```python
from build123d import *

# Parameters (mm, degrees)
SKETCH_1_R               = 37.5
EXTRUDE_1_DEPTH          = 7.5
SKETCH_2_R               = 2.05
CUT_EXTRUDE_1_DEPTH      = 54.560713214
CUT_EXTRUDE_2_DEPTH      = 3
PATTERN_CIRCULAR_1_COUNT = 4
SKETCH_4_R               = 3.05
CUT_EXTRUDE_3_DEPTH      = 4.5
PATTERN_CIRCULAR_2_COUNT = 6
SKETCH_7_R               = 28.2
SKETCH_7_R_2             = 21
CUT_EXTRUDE_4_DEPTH      = 4
SKETCH_9_R               = 6
CUT_EXTRUDE_5_DEPTH      = 54.560713214
EXTRUDE_3_DEPTH          = 4
FILLET_1_R               = 3
FILLET_3_R               = 3
FILLET_5_R               = 3.5
FILLET_6_R               = 3.5


with BuildPart() as part:
    # 草图1 → 凸台-拉伸1 (new body)
    with BuildSketch(Plane(origin=(0, 0, 0), x_dir=(1, 0, 0), z_dir=(0, 1, 0))):
        with Locations(Location((0, 0, 0), (0, 0, 270))):
            Circle(SKETCH_1_R)
    extrude(amount=EXTRUDE_1_DEPTH)

    # 草图2 → 切除-拉伸1 (cut, through all)
    with BuildSketch(Plane(origin=(0, 7.5, 0), x_dir=(1, 0, 0), z_dir=(0, 1, 0))):
        with Locations(Location((-31.5, 0, 0), (0, 0, 270))):
            Circle(SKETCH_2_R)
    cut_extrude_1 = extrude(amount=-CUT_EXTRUDE_1_DEPTH, mode=Mode.SUBTRACT)

    # 草图3 → 切除-拉伸2 (cut)
    with BuildSketch(Plane(origin=(0, 7.5, 0), x_dir=(1, 0, 0), z_dir=(0, 1, 0))):
        Polygon((-31.5, 3.944), (-34.915604193, 1.972), (-34.915604193, -1.972), (-31.5, -3.944), (-28.084395807, -1.972), (-28.084395807, 1.972), align=None)
    cut_extrude_2 = extrude(amount=-CUT_EXTRUDE_2_DEPTH, mode=Mode.SUBTRACT)

    # 阵列(圆周)1: 切除-拉伸1, 切除-拉伸2 ×4 about axis
    pattern_circular_1_axis = Axis((0, 0, 0), (0, 1, 0))
    add([cut_extrude_1.rotate(pattern_circular_1_axis, i * 360 / PATTERN_CIRCULAR_1_COUNT) for i in range(1, PATTERN_CIRCULAR_1_COUNT)], mode=Mode.SUBTRACT)
    add([cut_extrude_2.rotate(pattern_circular_1_axis, i * 360 / PATTERN_CIRCULAR_1_COUNT) for i in range(1, PATTERN_CIRCULAR_1_COUNT)], mode=Mode.SUBTRACT)

    # 草图4 → 切除-拉伸3 (cut)
    with BuildSketch(Plane.XZ):
        with Locations(Location((-13.5, 0, 0), (0, 0, 270))):
            Circle(SKETCH_4_R)
    cut_extrude_3 = extrude(amount=-CUT_EXTRUDE_3_DEPTH, mode=Mode.SUBTRACT)

    # 草图6 → CSK for M3 Countersunk Flat Head Screw1 (revolve, cut)
    with BuildSketch(Plane(origin=(-13.5, 4.5, 0), x_dir=(0, 0, -1), z_dir=(1, 0, 0))):
        Polygon((0, 0), (0, 3), (1.54, 3), (1.54, 1.48), (3.02, 0), align=None)
    csk_for_m3_countersunk_flat_head_screw1 = revolve(axis=Axis((-13.5, -1.85, 0), (0, 1, 0)), mode=Mode.SUBTRACT)

    # 阵列(圆周)2: 切除-拉伸3, CSK for M3 Countersunk Flat Head Screw1 ×6 about axis
    pattern_circular_2_axis = Axis((0, 0, 0), (0, 1, 0))
    add([cut_extrude_3.rotate(pattern_circular_2_axis, i * 360 / PATTERN_CIRCULAR_2_COUNT) for i in range(1, PATTERN_CIRCULAR_2_COUNT)], mode=Mode.SUBTRACT)
    add([csk_for_m3_countersunk_flat_head_screw1.rotate(pattern_circular_2_axis, i * 360 / PATTERN_CIRCULAR_2_COUNT) for i in range(1, PATTERN_CIRCULAR_2_COUNT)], mode=Mode.SUBTRACT)

    # 草图7 → 切除-拉伸4 (cut)
    with BuildSketch(Plane(origin=(0, 7.5, 0), x_dir=(1, 0, 0), z_dir=(0, 1, 0))):
        with Locations(Location((0, 0, 0), (0, 0, 270))):
            Circle(SKETCH_7_R)
        with Locations(Location((0, 0, 0), (0, 0, 270))):
            Circle(SKETCH_7_R_2, mode=Mode.SUBTRACT)
    extrude(amount=-CUT_EXTRUDE_4_DEPTH, mode=Mode.SUBTRACT)

    # 草图9 → 切除-拉伸5 (cut, through all)
    with BuildSketch(Plane(origin=(0, 7.5, 0), x_dir=(1, 0, 0), z_dir=(0, 1, 0))):
        with Locations(Location((0, 0, 0), (0, 0, 270))):
            Circle(SKETCH_9_R)
    extrude(amount=-CUT_EXTRUDE_5_DEPTH, mode=Mode.SUBTRACT)

    # 草图11 → 凸台-拉伸3 (add)
    with BuildSketch(Plane(origin=(0, 3.5, 0), x_dir=(1, 0, 0), z_dir=(0, 1, 0))):
        Polygon((-35.608419575, -11.759696227), (-36.717644054, -7.620014114), (-20.56188067, -4.267207904), (-19.940714962, -6.585429887), align=None)
    extrude(amount=EXTRUDE_3_DEPTH)

    # 圆角1
    # the kernel refuses this fillet: 3 mm, written as the material it takes off along each edge
    with BuildSketch(Plane(origin=(0, 7.5, 0), x_dir=(-0.9495578553408984, 0, 0.31359189938579934), z_dir=(-0.31359189938579934, 0, -0.9495578553408984))) as fillet_1_piece_1:
        with BuildLine():
            CenterArc((37.5 - FILLET_1_R, -FILLET_1_R), FILLET_1_R, 0, 90)
            Line((37.5 - FILLET_1_R, 0), (37.5, 0))
            Line((37.5, 0), (37.5, -FILLET_1_R))
        make_face()
    revolve(axis=Axis((0, 7.5, 0), (0, 1, 0)), revolution_arc=71.72417104, mode=Mode.SUBTRACT)
    with BuildSketch(Plane(origin=(0, 7.5, 0), x_dir=(-0.9791371747811866, 0, 0.20320037638133454), z_dir=(-0.20320037638133454, 0, -0.9791371747811866))) as fillet_1_piece_2:
        with BuildLine():
            CenterArc((37.5 - FILLET_1_R, -FILLET_1_R), FILLET_1_R, 0, 90)
            Line((37.5 - FILLET_1_R, 0), (37.5, 0))
            Line((37.5, 0), (37.5, -FILLET_1_R))
        make_face()
    revolve(axis=Axis((0, 7.5, 0), (0, 1, 0)), revolution_arc=6.55165792, mode=Mode.SUBTRACT)
    with BuildSketch(Plane(origin=(0, 7.5, 0), x_dir=(0, 0, 1), z_dir=(-1, 0, 0))) as fillet_1_piece_3:
        with BuildLine():
            CenterArc((37.5 - FILLET_1_R, -FILLET_1_R), FILLET_1_R, 0, 90)
            Line((37.5 - FILLET_1_R, 0), (37.5, 0))
            Line((37.5, 0), (37.5, -FILLET_1_R))
        make_face()
    revolve(axis=Axis((0, 7.5, 0), (0, 1, 0)), revolution_arc=281.72417104, mode=Mode.SUBTRACT)

    # 圆角3
    fillet_3_edges = [part.edges().sort_by_distance(p)[0] for p in [
        (0, 7.5, -6),
    ]]
    fillet(fillet_3_edges, radius=FILLET_3_R)

    # 圆角5
    fillet_5_edges = [part.edges().sort_by_distance(p)[0] for p in [
        (-26.777531521, 5.5, 8.843291563),
        (-27.611668329, 5.5, 5.730250614),
    ]]
    fillet(fillet_5_edges, radius=FILLET_5_R)

    # 圆角6
    fillet_6_edges = [part.edges().sort_by_distance(p)[0] for p in [
        (-20.56188067, 5.5, 4.267207904),
        (-19.940714962, 5.5, 6.585429887),
    ]]
    fillet(fillet_6_edges, radius=FILLET_6_R)


solid = part.part
```
Read the model definition and answer for the solid it produces. Units are mm, in the model's axes. A direction names the side the tool comes from. Give positions to 0.01 mm unless a question says otherwise; leave off trailing zeros. One line per item, written item: value. Start each with the question number.
(1) Flat-ended cylindrical pins translate along their axes: P1, Ø1.5, axis at x = 19.5, y = 3, coming from the -Z side; P2, Ø1.5, axis at x = -25.5, y = 3, coming from the +Z side; P3, Ø1, axis at y = 1.5, z = -0.5, coming from the -X side. Find the tip coordinate at first contact, or state that the pin passes through.
(2) For a pull along Z with two mould halves and no side action, classify faces 4 (the cylindrical face through (-22.818, 2.218, -29.759)), 5 (the cylindrical face through (-25.366, 5.528, 9.682)) as released by +Z, released by -Z, zero draft, split by the parting line, or undercut.
(3) Straight lines are drawn through the part: L1, parallel to X at y = 2.55, z = 0; L2, parallel to X at y = 6.75, z = -5; L3, parallel to X at y = 4.25, z = -18.5. For each, find the intervals that lie inside material, in ascending order.
(4) A tool of negligible diameter and unlimited length cuts with its end or side. For faces 1 (the flat face through (2.957, 6.021, -29.791)), 2 (the cylindrical face through (-12.134, 6.729, -0.711)), 3 (the cylindrical face through (-10.93, 2.22, -1.64)), from which of +Z, -Z, +X, -X, +Y, -Y can it reach the whole face along a straight path? Write none if from no direction.
(5) The part is cut by section A-A (z = 0). State how many separate pieces and enclosed holes the cut face has, and give its area (3 significant figures).
Taken from the geometry:
1. P1: z = -32.48
1. P2: z = 28.17
1. P3: x = -37.5
2. face 4: split by the parting line
2. face 5: undercut
3. L1: -37.5 to -33.55, -29.45 to -16.55, -10.45 to -6, 6 to 10.45, 16.55 to 29.45, 33.55 to 37.5
3. L2: -36.14 to -27.75, -20.4 to -4.92, 4.92 to 20.4, 27.75 to 36.14
3. L3: -32.62 to -21.28, -9.94 to 9.94, 21.28 to 32.62
4. face 1: +Y
4. face 2: +Y, -Y
4. face 3: -Y
5. separate pieces: 6
5. enclosed holes: 0
5. area: 252 mm^2
